Could you check a few things on this model? Use its own coordinates, in mm. Face numbers are marked on the shaded views. A direction names the side the tool comes from. Coordinates: 2 decimals unless noted, no trailing zeros. Order: outer loops, then holes, each group sorted by start corner. A loop starts at its lowest first (then second) coordinate and runs counter-clockwise, first axis right, second up. Notation, with made-up numbers: (4.5, 70.25) - (10.5, 70.25) arc R24 ccw to (10.5, 109.25) - close; hole circle Ø5 at (35.5, 54). An arc over 180 degrees is marked (long way). One line per item, written item: value. Start each with the question number.
from build123d import *

# Parameters (mm, degrees)
SKETCH1_W           = 10
SKETCH1_H           = 5
BOSS_EXTRUDE1_DEPTH = 3
FILLET1_R           = 2
SKETCH3_R           = 6.5
BOSS_EXTRUDE2_DEPTH = 2.5
SKETCH4_R           = 4.75
CUT_EXTRUDE1_DEPTH  = 6
SKETCH7_R           = 1.05
CUT_EXTRUDE2_DEPTH  = 2
BOSS_EXTRUDE3_DEPTH = 5


with BuildPart() as part:
    # Sketch1 → Boss-Extrude1 (new body)
    with BuildSketch(Plane.XY):
        Rectangle(SKETCH1_W, SKETCH1_H)
    extrude(amount=BOSS_EXTRUDE1_DEPTH)

    # Fillet1
    fillet1_edges = [part.edges().sort_by_distance(p)[0] for p in [
        (5, 2.5, 1.5),
        (5, -2.5, 1.5),
    ]]
    fillet(fillet1_edges, radius=FILLET1_R)

    # Sketch7 → Cut-Extrude2 (cut)
    with BuildSketch(Plane.XY.offset(3)):
        Circle(SKETCH7_R)
    extrude(amount=-CUT_EXTRUDE2_DEPTH, mode=Mode.SUBTRACT)



with BuildPart() as body_2:
    # Sketch3 → Boss-Extrude2 (new body, symmetric)
    with BuildSketch(Plane(origin=(0, 0, 0), x_dir=(1, 0, 0), z_dir=(0, 1, 0))):
        with Locations((-9.8, -0.5)):
            Circle(SKETCH3_R)
    extrude(amount=BOSS_EXTRUDE2_DEPTH, both=True)

    # Sketch4 → Cut-Extrude1 (cut, through all)
    with BuildSketch(Plane.XZ.offset(2.5)):
        with Locations((-9.8, 0.5)):
            Circle(SKETCH4_R)
    extrude(amount=-CUT_EXTRUDE1_DEPTH, mode=Mode.SUBTRACT)


with BuildPart() as part_1:
    add(part.part)

    add(body_2.part)  # Boss-Extrude3 merges body 2
    # Sketch8 → Boss-Extrude3 (add)
    with BuildSketch(Plane.XZ.offset(2.5)):
        with BuildLine():
            Line((-5.77711019, 5.605522263), (-2.470394732, 3))
            Line((-2.470394732, 3), (-3.8, 3))
            ThreePointArc((-3.8, 3), (-4.621992024, 4.42915174), (-5.77711019, 5.605522263))
        make_face()
        with BuildLine():
            Line((-5.748087743, -4.582519755), (0, 0))
            Line((0, 0), (-3.319259302, 0))
            ThreePointArc((-3.319259302, 0), (-4.056824363, -2.543999606), (-5.748087743, -4.582519755))
        make_face()
    extrude(amount=-BOSS_EXTRUDE3_DEPTH)


solid = part_1.part
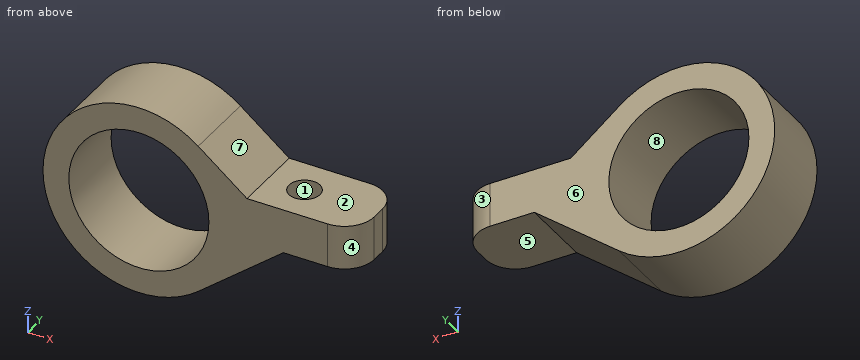
Q1. Which directions (+Z, -Z, +X, -X, +Y, -Y) give clear straight access to the entire face, cutting with the end or side of a thin tool? Please do the marked faces 1, 2, 3, 4 and 5.
Q2. I want a section at B-B on z = 0.5. Please give me the cut outline in (x, y), then the cut area to 3 significant figures.
Q3. I want a section at D-D on x = -7.5. Please give me the cut outline in (y, z), then the cut area to 3 significant figures.
Q4. If I drill on L1, parallel to Z at x = -9.8, y = -0.45; L2, parallel to Y at x = 0, z = 1.65; L3, parallel to Z at x = 4, y = 2.15, over which ranges is the centre line in solid material (lowest first)?
Q5. I want a section at C-C on y = 2. Please give me the cut outline in (x, z).
Q6. I'm going to push flat-ended pins straight in: pin 1 (3 mm diameter, centred on y = -1, z = -2, fed in from +X); pin 2 (2.5 mm diameter, centred on x = 0, y = 0.5, fed in from +Z); pin 3 (1.5 mm diameter, centred on x = 2, y = 1.5, fed in from -Z). Where does each tip first touch, or does it pass through?
Q7. We'd pull the mould along Z, two halves only. Please class the marked faces 6, 7 and 8: +Z half, -Z half, draft (parallel to the pull), parting line (faces both ways), or undercut.
Q8. I want a section at A-A on x = -9.8. Please give me the cut outline in (y, z), then the cut area to 3 significant figures.
Values follow:
1. face 1: +Z
1. face 2: +Z, +X, +Y, -Y
1. face 3: +Z, -Z, +X, +Y
1. face 4: +Z, -Z, +X, -Y
1. face 5: -Z, +X, +Y, -Y
2. outline: (-16.3, -2.5) - (-14.55, -2.5) - (-14.55, 2.5) - (-16.3, 2.5) - close; (-5.05, -2.5) - (3, -2.5) arc R2 ccw to (5, -0.5) - (5, 0.5) arc R2 ccw to (3, 2.5) - (-5.05, 2.5) - close
2. area: 57.3 mm^2
3. outline: (-2.5, -5.58) - (2.5, -5.58) - (2.5, -3.66) - (-2.5, -3.66) - close; (-2.5, 4.66) - (2.5, 4.66) - (2.5, 6.58) - (-2.5, 6.58) - close
3. area: 19.2 mm^2
4. L1: z = -6 to -4.25, 5.25 to 7
4. L2: y = -2.5 to -1.05, 1.05 to 2.5
4. L3: z = 0 to 3
5. outline: (-5.78, 5.61) arc R6.5 ccw (long way) to (-5.75, -4.58) - (0, 0) - (4.32, 0) - (4.32, 3) - (-2.47, 3) - close; hole circle Ø9.5 at (-9.8, 0.5)
6. pin 1: stops at x = -0.63
6. pin 2: stops at z = 3
6. pin 3: stops at z = 0
7. face 6: draft
7. face 7: +Z half
7. face 8: undercut
8. outline: (-2.5, -6) - (2.5, -6) - (2.5, -4.25) - (-2.5, -4.25) - close; (-2.5, 5.25) - (2.5, 5.25) - (2.5, 7) - (-2.5, 7) - close
8. area: 17.5 mm^2
